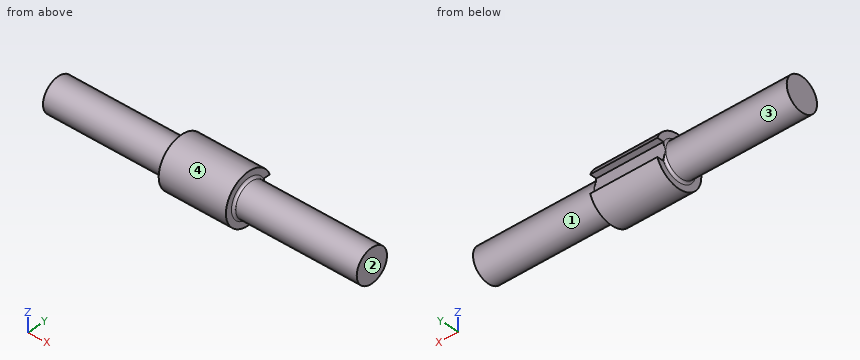
from build123d import *

# Parameters (mm, degrees)
CUT_EXTRUDE1_DEPTH      = 72.785270077
CUT_EXTRUDE1_DEPTH_BACK = 72.785270077
SKETCH4_W               = 4
SKETCH4_H               = 3
FILLET5_R               = 1
FILLET6_R               = 1


with BuildPart() as part:
    # Sketch1 → Revolve1 (revolve)
    with BuildSketch(Plane.XY, mode=Mode.PRIVATE) as revolve1_sk:
        Polygon((0, 0), (70, 0), (70, 7.5), (15, 7.5), (15, 11.25), (-15, 11.25), (-15, 7.5), (-70, 7.5), (-70, 0), align=None)
    revolve(revolve1_sk.sketch.rotate(Axis((0, 0, 0), (1, 0, 0)), 90), axis=Axis((0, 0, 0), (1, 0, 0)))

    # Sketch4 → Cut-Extrude1 (cut, two sides: drawn at the far end of the back side and taken through both)
    with BuildSketch(Plane(origin=(0, 0, 0), x_dir=(0, 0, -1), z_dir=(1, 0, 0)).offset(-CUT_EXTRUDE1_DEPTH_BACK)):
        with Locations((2, 9.014870422)):
            Rectangle(SKETCH4_W, SKETCH4_H)
        with Locations((-2, 9.014870422)):
            Rectangle(SKETCH4_W, SKETCH4_H)
        with BuildLine():
            Line((0, 11.25), (0, 10.514870422))
            Line((0, 10.514870422), (4, 10.514870422))
            ThreePointArc((4, 10.514870422), (2.033495482, 11.064691416), (0, 11.25))
        make_face()
        with BuildLine():
            Line((-4, 10.514870422), (0, 10.514870422))
            Line((0, 10.514870422), (0, 11.25))
            ThreePointArc((0, 11.25), (-2.033495482, 11.064691416), (-4, 10.514870422))
        make_face()
    extrude(amount=CUT_EXTRUDE1_DEPTH + CUT_EXTRUDE1_DEPTH_BACK, mode=Mode.SUBTRACT)

    # Fillet5
    # the kernel refuses this fillet: 1 mm, written as the material it adds along each edge
    with BuildSketch(Plane(origin=(-15, 0, 0), x_dir=(0, 0, 1), z_dir=(0, 1, 0))) as fillet5_piece_1_section:
        with BuildLine():
            CenterArc((7.5 + FILLET5_R, -FILLET5_R), FILLET5_R, 90, 90)
            Line((7.5, -FILLET5_R), (7.5, 0))
            Line((7.5, 0), (7.5 + FILLET5_R, 0))
        make_face()
    fillet5_piece_1 = revolve(axis=Axis((-15, 0, 0), (1, 0, 0)), mode=Mode.PRIVATE)
    fillet5_piece_1 = split(fillet5_piece_1, bisect_by=Plane(origin=(-15.276890307, 7.514870422, -7.776890307), z_dir=(0, -1, 0)), keep=Keep.TOP, mode=Mode.PRIVATE)
    add(fillet5_piece_1)

    # Fillet6
    # the kernel refuses this fillet: 1 mm, written as the material it adds along each edge
    with BuildSketch(Plane(origin=(15, 0, 0), x_dir=(0, 0, 1), z_dir=(0, 1, 0))) as fillet6_piece_1_section:
        with BuildLine():
            CenterArc((7.5 + FILLET6_R, FILLET6_R), FILLET6_R, 180, 90)
            Line((7.5, FILLET6_R), (7.5, 0))
            Line((7.5, 0), (7.5 + FILLET6_R, 0))
        make_face()
    fillet6_piece_1 = revolve(axis=Axis((15, 0, 0), (1, 0, 0)), mode=Mode.PRIVATE)
    fillet6_piece_1 = split(fillet6_piece_1, bisect_by=Plane(origin=(15.276890307, 7.514870422, -7.776890307), z_dir=(0, -1, 0)), keep=Keep.TOP, mode=Mode.PRIVATE)
    add(fillet6_piece_1)


solid = part.part
Could you check a few things on this model? Use its own coordinates, in mm. Face numbers are marked on the shaded views. A direction names the side the tool comes from. Coordinates: 2 decimals unless noted, no trailing zeros. Order: outer loops, then holes, each group sorted by start corner. A loop starts at its lowest first (then second) coordinate and runs counter-clockwise, first axis right, second up.
Q1. Suppose I cut it at D-D on x = 54. Please give me the cut outline in (y, z), and give its area (3 significant figures).
Q2. Will these pins go through, and if not, where does the flat tip stop? pin 1 (8 mm diameter, centred on x = 37.5, y = 2.5, fed in from +Z); pin 2 (1.5 mm diameter, centred on x = 1.5, y = 9.5, fed in from +Z); pin 3 (3 mm diameter, centred on x = 39.5, y = 3.5, fed in from +Z); pin 4 (10 mm diameter, centred on x = 7, y = -3, fed in from +Z).
Q3. Thinking about a two-plate mould opening in Y: for the marked faces 1 and 2, which applies, released by +Y, released by -Y, zero draft, split by the parting line, or undercut?
Q4. Please list where these lines run through material, in increasing order: L1, parallel to X at y = 7, z = -7.25; L2, parallel to Z at x = -10, y = 0.25; L3, parallel to Z at x = 40, y = 2.25.
Q5. Suppose I cut it at B-B on z = 0. Please give me the cut outline in (x, y).
Q6. Suppose I cut it at C-C on x = 8. Please give me the cut outline in (y, z), and give its area (3 significant figures).
Q7. Suppose I cut it at A-A on y = 0. Please give me the cut outline in (x, z), and give its area (3 significant figures).
Q8. Which directions (+Z, -Z, +X, -X, +Y, -Y) give clear straight access to the entire face, cutting with the end or side of a thin tool? Please do the marked faces 3 and 4.
Answer:
1. outline: circle Ø15 at (0, 0)
1. area: 177 mm2
2. pin 1: stops at z = 7.5
2. pin 2: stops at z = 7.07
2. pin 3: stops at z = 7.23
2. pin 4: stops at z = 11.25
3. face 1: split by the parting line
3. face 2: zero draft
4. L1: x = -15 to 15
4. L2: z = -11.25 to 11.25
4. L3: z = -7.15 to 7.15
5. outline: (-70, -7.5) - (-16, -7.5) arc R1 cw to (-15, -8.5) - (-15, -11.25) - (15, -11.25) - (15, -8.5) arc R1 cw to (16, -7.5) - (70, -7.5) - (70, 7.5) - (16, 7.5) arc R1 cw to (15.83, 7.51) - (-15.83, 7.51) arc R1 cw to (-16, 7.5) - (-70, 7.5) - close
6. outline: (7.51, -4) - (7.51, 4) - (10.51, 4) arc R11.25 ccw (long way) to (10.51, -4) - close
6. area: 370 mm2
7. outline: (-70, -7.5) - (-16, -7.5) arc R1 cw to (-15, -8.5) - (-15, -11.25) - (15, -11.25) - (15, -8.5) arc R1 cw to (16, -7.5) - (70, -7.5) - (70, 7.5) - (16, 7.5) arc R1 cw to (15, 8.5) - (15, 11.25) - (-15, 11.25) - (-15, 8.5) arc R1 cw to (-16, 7.5) - (-70, 7.5) - close
7. area: 2,330 mm2
8. face 3: -X
8. face 4: +X, -X
